from build123d import *

# Parameters (mm, degrees)
SKETCH1_R           = 4
BOSS_EXTRUDE1_DEPTH = 100
SKETCH2_W           = 1
SKETCH2_H           = 0.8
SKETCH3_W           = 1
SKETCH3_H           = 0.8
LPATTERN1_COUNT     = 2
LPATTERN1_PITCH     = 18


with BuildPart() as part:
    # Sketch1 → Boss-Extrude1 (new body)
    with BuildSketch(Plane(origin=(0, 0, 0), x_dir=(1, 0, 0), z_dir=(0, 1, 0))):
        with Locations(Location((0, 0, 0), (0, 0, 270))):
            Circle(SKETCH1_R)
    extrude(amount=BOSS_EXTRUDE1_DEPTH)

    # Sketch2 → Cut-Revolve1 (revolve, cut)
    with BuildSketch(Plane(origin=(0, 0, 0), x_dir=(0, 0, -1), z_dir=(1, 0, 0)), mode=Mode.PRIVATE) as cut_revolve1_sk:
        with Locations((3.5, 97.4)):
            Rectangle(SKETCH2_W, SKETCH2_H)
    revolve(cut_revolve1_sk.sketch.rotate(Axis((0, 100, 0), (0, -1, 0)), 180), axis=Axis((0, 100, 0), (0, -1, 0)), mode=Mode.SUBTRACT)

    # Sketch3 → Cut-Revolve2 (revolve, cut)
    with BuildSketch(Plane(origin=(0, 0, 0), x_dir=(0, 0, -1), z_dir=(1, 0, 0)), mode=Mode.PRIVATE) as cut_revolve2_sk:
        with Locations((3.5, 60.1)):
            Rectangle(SKETCH3_W, SKETCH3_H)
    cut_revolve2 = revolve(cut_revolve2_sk.sketch.rotate(Axis((0, 100, 0), (0, -1, 0)), 180), axis=Axis((0, 100, 0), (0, -1, 0)), mode=Mode.SUBTRACT)

    # LPattern1: Cut-Revolve2 ×2
    with Locations(*[(0, -i * LPATTERN1_PITCH, 0) for i in range(1, LPATTERN1_COUNT)]):
        add(cut_revolve2, mode=Mode.SUBTRACT)


solid = part.part
Read the model definition and answer for the solid it produces. Units are mm, in the model's axes. A direction names the side the tool comes from. Give positions to 0.01 mm unless a question says otherwise; leave off trailing zeros. Loops run counter-clockwise (first coordinate to the right, second up) from the corner with the lowest first, then second, coordinate; pieces in that order, holes last. Notation, with made-up numbers: (14, 43) -> (47, 43) arc R9 cw to (47, 55) -> close; hole circle Ø4 at (39.25, 14). An arc over 180 degrees is marked (long way). Use a Markdown table: item, result.
Q1. This flat-tipped pin is pushed along its axis until it touches: pin 1 (1 mm diameter, centred on y = 39.5, z = 2, fed in from +X). Where does it stop, or does it pass through?
Solved:
| item | result |
|---|---|
| pin 1 | stops at x = 3.71 |
Q2. A tool of negligible diameter and unlimited length cuts with its end or side. For faces 1 (the face through (-3.905, 20.558, -0.867)), 2 (the face through (-3, 97, -1)), from which of +Z, -Z, +X, -X, +Y, -Y can it reach the whole face along a straight path? Write none if from no direction.
Solved:
| item | result |
|---|---|
| face 1 | +Y, -Y |
| face 2 | none |
Q3. Section A-A, the plane z = 1.25 is taken. Determine the outline of the cut face in (x, y).
Solved:
| item | result |
|---|---|
| outline | (-3.8, 0) -> (3.8, 0) -> (3.8, 41.7) -> (2.73, 41.7) -> (2.73, 42.5) -> (3.8, 42.5) -> (3.8, 59.7) -> (2.73, 59.7) -> (2.73, 60.5) -> (3.8, 60.5) -> (3.8, 97) -> (2.73, 97) -> (2.73, 97.8) -> (3.8, 97.8) -> (3.8, 100) -> (-3.8, 100) -> (-3.8, 97.8) -> (-2.73, 97.8) -> (-2.73, 97) -> (-3.8, 97) -> (-3.8, 60.5) -> (-2.73, 60.5) -> (-2.73, 59.7) -> (-3.8, 59.7) -> (-3.8, 42.5) -> (-2.73, 42.5) -> (-2.73, 41.7) -> (-3.8, 41.7) -> close |
Q4. Determine the mould class of faces 3 (the face through (-0.9, 60.11, 2.86)), 4 (the face through (-3.905, 78.494, -0.867)), 5 (the face through (0, 0, 0)) for opening direction Y: pulls with the +Y half, pulls with the -Y half, needs draft (parallel to the pull), parting line crosses it, or undercut.
Solved:
| item | result |
|---|---|
| face 3 | undercut |
| face 4 | needs draft |
| face 5 | pulls with the -Y half |
Q5. Find the intervals of material crossed by line 1 along Y through (x, z) = (1.75, 3.5); line 2 along Z through (x, y) = (0.25, 18); line 3 along X through (y, z) = (58, 2.5), in increasing order.
Solved:
| item | result |
|---|---|
| line 1 | y = 0 to 41.7, 42.5 to 59.7, 60.5 to 97, 97.8 to 100 |
| line 2 | z = -3.99 to 3.99 |
| line 3 | x = -3.12 to 3.12 |
Q6. Section B-B, the plane y = 74.5 is taken. Determine the outline of the cut face in (x, z).
Solved:
| item | result |
|---|---|
| outline | circle Ø8 at (0, 0) |
